Can you work these out from the model? Positions are in its coordinate system, mm. A direction names the side the tool comes from. Coordinates: 2 decimals unless noted, no trailing zeros. Write each loop counter-clockwise with the first axis right and the second up, starting at its lowest first coordinate (ties: lowest second). Pieces come first, ordered by that corner, then holes. Notation, with made-up numbers: (28, 62.5) -> (39, 62.5) arc R15 cw to (39, 81.5) -> close; hole circle Ø6 at (77, -29). An arc over 180 degrees is marked (long way). Use one line per item in the form item = value.
```python
from build123d import *

# Parameters (mm, degrees)
F3_R     = 4.7700695271
F4_DEPTH = 25.908
F5_R     = 7.5557207763
F6_DEPTH = 24.638
F7_R     = 8.9716016728
F7_R_2   = 7.5557207763
F8_DEPTH = 3.302


# Not quite as in the source:
# - a feature names something its author has since deleted; it is built from what else it names


with BuildPart() as f2:
    # F0 (on Top) → F2 (revolve)
    with BuildSketch(Plane.XY):
        with BuildLine():
            Line((0, 24.6944446117), (0, -24.6944446117))
            ThreePointArc((0, -24.6944446117), (16.6301779866, -18.2552122643), (24.5875081551, -2.2956562028))
            Line((24.5875081551, -2.2956562028), (23.6113984138, -2.2956562028))
            Line((23.6113984138, -2.2956562028), (23.6113984138, 2.2956562028))
            Line((23.6113984138, 2.2956562028), (24.5875081551, 2.2956562028))
            ThreePointArc((24.5875081551, 2.2956562028), (16.6301779866, 18.2552122643), (0, 24.6944446117))
        make_face()
    revolve(axis=Axis((0, 0.329259783, 0), (0, -1, 0)))

    # F3 (on Top) → F4 (join)
    with BuildSketch(Plane.XY):
        Circle(F3_R)
    extrude(amount=F4_DEPTH)

    # F5 (on Top) → F6 (join)
    with BuildSketch(Plane.XY):
        Circle(F5_R)
    extrude(amount=F6_DEPTH)

    # F7 (on face) → F8 (cut)
    with BuildSketch(Plane.XY.offset(24.638)):
        Circle(F7_R)
        Circle(F7_R_2, mode=Mode.SUBTRACT)
    extrude(amount=-F8_DEPTH, mode=Mode.SUBTRACT)


solid = f2.part
```
Q1. Will these pins go through, and if not, where does the flat tip stop? pin 1 (3 mm diameter, centred on x = -2.5, z = -0.5, fed in from +Y); pin 2 (23.5 mm diameter, centred on x = 0, y = 0, fed in from -Z); pin 3 (10 mm diameter, centred on y = 19.5, z = 18.5, fed in from -X); pin 4 (12 mm diameter, centred on x = -13, y = 11, fed in from +Z).
Return value:
pin_1 = 24.67
pin_2 = -24.59
pin_3 = -11.45
pin_4 = 22.09
Q2. If I drill on line 1 (Y direction, x = 0, z = 22.05); line 2 (Y direction, x = 0, z = 21.8); line 3 (X direction, y = -1.5, z = 5), over which ranges is the centre line in solid material (lowest first)? Write a range as from..to.
Return value:
line_1 = -11.12..-8.97, -7.56..7.56, 8.97..11.12
line_2 = -11.6..-8.97, -7.56..7.56, 8.97..11.6
line_3 = -23.08..23.08
Q3. Suppose I cut it at D-D (z = -6). Write out the boundary of the cut face in (x, y).
Return value:
outline = (-23.84, -2.3) arc R23.95 ccw to (23.84, -2.3) -> (22.84, -2.3) -> (22.84, 2.3) -> (23.84, 2.3) arc R23.95 ccw to (-23.84, 2.3) -> (-22.84, 2.3) -> (-22.84, -2.3) -> close
Q4. Suppose I cut it at C-C (y = 5.5). Write out the boundary of the cut face in (x, z).
Return value:
outline = (-7.09, 21.34) -> (-7.09, 23.01) arc R24.07 ccw (long way) to (7.09, 23.01) -> (7.09, 21.34) -> (5.18, 21.34) -> (5.18, 24.64) -> (-5.18, 24.64) -> (-5.18, 21.34) -> close
Q5. Suppose I cut it at A-A (x = 0). Write out the boundary of the cut face in (y, z).
Return value:
outline = (-8.97, 21.34) -> (-8.97, 23.01) arc R24.69 ccw to (-2.3, -24.59) -> (-2.3, -23.61) -> (2.3, -23.61) -> (2.3, -24.59) arc R24.69 ccw to (8.97, 23.01) -> (8.97, 21.34) -> (7.56, 21.34) -> (7.56, 24.64) -> (4.77, 24.64) -> (4.77, 25.91) -> (-4.77, 25.91) -> (-4.77, 24.64) -> (-7.56, 24.64) -> (-7.56, 21.34) -> close
Q6. For faces 4 (the flat face through (0, -5, 24.638)), 5 (the flat face through (-2, 2.296, -24)), which set-ups out of +Z, -Z, +X, -X, +Y, -Y let a thin tool reach every point of the face, with its end or its side?
Return value:
face_4 = +Z
face_5 = none
Q7. Thinking about a two-plate mould opening in Y: for faces 1 (the flat face through (0, 0, 25.908)), 2 (the cylindrical face through (-1.034, -4.657, 25.264)), 3 (the cylindrical face through (-0.914, 0.032, -23.594)), which applies, released by +Y, released by -Y, zero draft, split by the parting line, or undercut?
Return value:
face_1 = zero draft
face_2 = split by the parting line
face_3 = undercut
